from build123d import *

# Parameters (mm, degrees)
SKETCH_1_W      = 220
SKETCH_1_H      = 381
SKETCH_1_W_2    = 139
SKETCH_1_H_2    = 285
EXTRUDE_1_DEPTH = 4


with BuildPart() as part:
    # 草圖1 → 填料-伸長1 (new body)
    with BuildSketch(Plane.XZ.offset(4)):
        with Locations((-3.755314961, -3.521610711)):
            Rectangle(SKETCH_1_W, SKETCH_1_H)
        with BuildLine():
            Line((-85.755314961, 152.478389289), (-85.755314961, -132.521610711))
            ThreePointArc((-85.755314961, -132.521610711), (-87.255314961, -134.021610711), (-88.755314961, -132.521610711))
            Line((-88.755314961, -132.521610711), (-88.755314961, 152.478389289))
            ThreePointArc((-88.755314961, 152.478389289), (-87.255314961, 153.978389289), (-85.755314961, 152.478389289))
        make_face(mode=Mode.SUBTRACT)
        with BuildLine():
            Line((-105.755314961, -122.521610711), (-107.755314961, -122.521610711))
            ThreePointArc((-107.755314961, -122.521610711), (-109.255314961, -121.021610711), (-107.755314961, -119.521610711))
            Line((-107.755314961, -119.521610711), (-105.755314961, -119.521610711))
            ThreePointArc((-105.755314961, -119.521610711), (-104.255314961, -121.021610711), (-105.755314961, -122.521610711))
        make_face(mode=Mode.SUBTRACT)
        with BuildLine():
            Line((98.244685039, 115.478389289), (100.244685039, 115.478389289))
            ThreePointArc((100.244685039, 115.478389289), (101.744685039, 113.978389289), (100.244685039, 112.478389289))
            Line((100.244685039, 112.478389289), (98.244685039, 112.478389289))
            ThreePointArc((98.244685039, 112.478389289), (96.744685039, 113.978389289), (98.244685039, 115.478389289))
        make_face(mode=Mode.SUBTRACT)
        with BuildLine():
            Line((98.244685039, -2.021610711), (100.244685039, -2.021610711))
            ThreePointArc((100.244685039, -2.021610711), (101.744685039, -3.521610711), (100.244685039, -5.021610711))
            Line((100.244685039, -5.021610711), (98.244685039, -5.021610711))
            ThreePointArc((98.244685039, -5.021610711), (96.744685039, -3.521610711), (98.244685039, -2.021610711))
        make_face(mode=Mode.SUBTRACT)
        with BuildLine():
            Line((-107.755314961, -2.021610711), (-105.755314961, -2.021610711))
            ThreePointArc((-105.755314961, -2.021610711), (-104.255314961, -3.521610711), (-105.755314961, -5.021610711))
            Line((-105.755314961, -5.021610711), (-107.755314961, -5.021610711))
            ThreePointArc((-107.755314961, -5.021610711), (-109.255314961, -3.521610711), (-107.755314961, -2.021610711))
        make_face(mode=Mode.SUBTRACT)
        with BuildLine():
            Line((-107.755314961, 115.478389289), (-105.755314961, 115.478389289))
            ThreePointArc((-105.755314961, 115.478389289), (-104.255314961, 113.978389289), (-105.755314961, 112.478389289))
            Line((-105.755314961, 112.478389289), (-107.755314961, 112.478389289))
            ThreePointArc((-107.755314961, 112.478389289), (-109.255314961, 113.978389289), (-107.755314961, 115.478389289))
        make_face(mode=Mode.SUBTRACT)
        with BuildLine():
            Line((98.244685039, -119.521610711), (100.244685039, -119.521610711))
            ThreePointArc((100.244685039, -119.521610711), (101.744685039, -121.021610711), (100.244685039, -122.521610711))
            Line((100.244685039, -122.521610711), (98.244685039, -122.521610711))
            ThreePointArc((98.244685039, -122.521610711), (96.744685039, -121.021610711), (98.244685039, -119.521610711))
        make_face(mode=Mode.SUBTRACT)
        with Locations((16.744685039, 9.978389289)):
            Rectangle(SKETCH_1_W_2, SKETCH_1_H_2, mode=Mode.SUBTRACT)
    extrude(amount=-EXTRUDE_1_DEPTH)


solid = part.part
Can you work these out from the model? Positions are in its coordinate system, mm. Round coordinates to 2 decimals unless told otherwise and drop trailing zeros. Write each loop counter-clockwise with the first axis right and the second up, starting at its lowest first coordinate (ties: lowest second). Pieces come first, ordered by that corner, then holes. Notation, with made-up numbers: (69, 88.25) - (75, 88.25) arc R13 ccw to (75, 97.25) - close; hole circle Ø4 at (-28, -0.75). An arc over 180 degrees is marked (long way). Write each question's results on one line, items separated by ' | '. Start each with the question number.
1) Suppose I cut it at C-C (y = -1.65). Give the number of separate pieces and of enclosed holes in the cut face, and give its area (3 significant figures).
2) Suppose I cut it at A-A (z = -58.5). List the corners of the cut face in (x, y) for me, and give its area (3 significant figures).
3) Please list where these lines run through material, in increasing order: line 1 (X direction, y = -2.75, z = -55); line 2 (Z direction, x = 17.5, y = -0.25).
4) Suppose I cut it at B-B (x = 14). List the corners of the cut face in (y, z) for me.
Here are the results:
1) separate pieces: 1 | enclosed holes: 8 | area: 43,300 mm2
2) outline: (-113.76, -4) - (-88.76, -4) - (-88.76, 0) - (-113.76, 0) - close; (-85.76, -4) - (-52.76, -4) - (-52.76, 0) - (-85.76, 0) - close; (86.24, -4) - (106.24, -4) - (106.24, 0) - (86.24, 0) - close | area: 312 mm2
3) line 1: x = -113.76 to -88.76, -85.76 to -52.76, 86.24 to 106.24 | line 2: z = -194.02 to -132.52, 152.48 to 186.98
4) outline: (-4, -194.02) - (0, -194.02) - (0, -132.52) - (-4, -132.52) - close; (-4, 152.48) - (0, 152.48) - (0, 186.98) - (-4, 186.98) - close
